from build123d import *

# Parameters (mm, degrees)
SKETCH1_W           = 4
SKETCH1_H           = 2
BOSS_EXTRUDE1_DEPTH = 3.5
WIRE_CANAL_DEPTH    = 1.5
SKETCH2_R           = 0.8
SCREW_HOLES_DEPTH   = 43.383720665
FILLET1_START       = 14.161255893
FILLET1_DEPTH       = 27.838744107
CUT_EXTRUDE1_START  = 3.5
SKETCH4_R           = 1.25
CUT_EXTRUDE1_DEPTH  = 3


with BuildPart() as part:
    # Sketch1 → Boss-Extrude1 (new body)
    with BuildSketch(Plane.XY):
        with BuildLine():
            Line((10.161255893, 0), (36.161255894, 0))
            ThreePointArc((36.161255894, 0), (37.476597455, 4.684658438), (41.038150268, 8))
            Line((41.038150268, 8), (14.161255893, 8))
            Line((14.161255893, 8), (10.161255893, 8))
            Line((10.161255893, 8), (10.161255893, 0))
        make_face()
        Polygon((36.161255894, -8), (36.161255894, 0), (10.161255893, 0), (10.161255893, -8), (14.161255893, -8), align=None)
        with Locations((12.161255893, 9)):
            Rectangle(SKETCH1_W, SKETCH1_H)
        with Locations((12.161255893, -9)):
            Rectangle(SKETCH1_W, SKETCH1_H)
    extrude(amount=BOSS_EXTRUDE1_DEPTH)

    # Sketch3 → Wire Canal (cut)
    with BuildSketch(Plane.XY):
        Polygon((10.161255893, 3), (10.161255893, 0), (10.161255893, -3), (38.287392351, -3), (38.287392351, 3), align=None)
    extrude(amount=WIRE_CANAL_DEPTH, mode=Mode.SUBTRACT)

    # Sketch2 → Screw Holes (cut, through all)
    with BuildSketch(Plane.XY):
        with Locations(Location((20.161255894, 0, 0), (0, 0, 180))):
            Circle(SKETCH2_R)
        with Locations((12.161255894, -6.25)):
            Circle(SKETCH2_R)
        with Locations((29.661255894, 6.25)):
            Circle(SKETCH2_R)
        with Locations((29.661255894, -6.25)):
            Circle(SKETCH2_R)
        with Locations((12.161255894, 6.25)):
            Circle(SKETCH2_R)
        with Locations(Location((28.161255894, 0, 0), (0, 0, 180))):
            Circle(SKETCH2_R)
    extrude(amount=SCREW_HOLES_DEPTH, mode=Mode.SUBTRACT)

    # Fillet1: read off the stored shape, not the designer's step
    # Fillet1 outline → Fillet1 (cut)
    with BuildSketch(Plane.YZ.offset(FILLET1_START)):
        with BuildLine():
            Line((-8, 3.5), (-8, 0.5))
            ThreePointArc((-8, 0.5), (-7.121320344, 2.621320344), (-5, 3.5))
            Line((-5, 3.5), (-8, 3.5))
        make_face()
        with BuildLine():
            Line((8, 3.5), (5, 3.5))
            ThreePointArc((5, 3.5), (7.121320344, 2.621320344), (8, 0.5))
            Line((8, 0.5), (8, 3.5))
        make_face()
    extrude(amount=FILLET1_DEPTH, mode=Mode.SUBTRACT)

    # Sketch4 → Cut-Extrude1 (cut)
    with BuildSketch(Plane.XY.offset(CUT_EXTRUDE1_START)):
        with Locations((29.661255894, -6.25)):
            Circle(SKETCH4_R)
    extrude(amount=-CUT_EXTRUDE1_DEPTH, mode=Mode.SUBTRACT)


solid = part.part
Source: CAD feature listing. Evaluate the final solid. Frame: model axes, mm. A direction names the side the tool comes from. Round coordinates to 2 decimals unless told otherwise and drop trailing zeros. Loops run counter-clockwise (first coordinate to the right, second up) from the corner with the lowest first, then second, coordinate; pieces in that order, holes last. Notation, with made-up numbers: M 4,-33 L 8,-33 A9 ccw 8,-19 Z; hole C 21.25,-11.5 d4. An arc over 180 degrees is marked long. Answer as CSV lines item,"result".
Q1. Contact query for flat-ended pins moving along their axis: pin 1 (1.8 mm diameter, centred on y = 7, z = 1.5, fed in from +X); pin 2 (1.4 mm diameter, centred on x = 29.66, y = 6.25, fed in from -Z); pin 3 (2 mm diameter, centred on x = 28.16, y = 0, fed in from -Z); pin 4 (1 mm diameter, centred on x = 32.5, z = 1.5, fed in from -Y). Output: stop coordinate, or through.
Verdict:
pin 1,"stops at x = 40.82"
pin 2,"passes through"
pin 3,"stops at z = 1.5"
pin 4,"stops at y = -7.96"
Q2. Cut plane A-A (x = 17). Return the cut outline in (y, z).
Verdict:
outline,"M -8,0 L -3,0 L -3,1.5 L 3,1.5 L 3,0 L 8,0 L 8,0.5 A3 ccw 5,3.5 L -5,3.5 A3 ccw -8,0.5 Z"
Q3. Cut plane D-D (y = -4.25). Return the cut outline in (x, z).
Verdict:
outline,"M 10.16,0 L 36.16,0 L 36.16,3.5 L 10.16,3.5 Z"
Q4. Cut plane B-B (y = 6.25). Return the cut outline in (x, z), plus the area to 3 significant figures.
Verdict:
outline,"M 10.16,0 L 11.36,0 L 11.36,3.5 L 10.16,3.5 Z; M 12.96,0 L 28.86,0 L 28.86,3.23 L 14.16,3.23 L 14.16,3.5 L 12.96,3.5 Z; M 30.46,0 L 38.69,0 L 38.69,3.23 L 30.46,3.23 Z"
area,"82.4 mm^2"
Q5. Reachability of faces 5 (the face through (36.161, -4, 2)), 6 (the face through (23, 0, 1.5)), 7 (the face through (11.57, 6.79, 1.73)) from +Z, -Z, +X, -X, +Y, -Y: full face, straight path, thin tool, end or side. Return the list, or none.
Verdict:
face 5,"+Z, -Z, +X, -Y"
face 6,"-Z, +X, -X"
face 7,"+Z, -Z"
Q6. Cut plane C-C (z = 2.85). Return the cut outline in (x, y), plus the area to 3 significant figures.
Verdict:
outline,"M 10.16,-10 L 14.16,-10 L 14.16,-6.86 L 28.57,-6.86 A1.25 cw long 30.75,-6.86 L 36.16,-6.86 L 36.16,0 A9 cw 39.34,6.86 L 30.17,6.86 A0.8 cw long 29.15,6.86 L 14.16,6.86 L 14.16,10 L 10.16,10 Z; hole C 12.16,-6.25 d1.6; hole C 12.16,6.25 d1.6; hole C 20.16,0 d1.6; hole C 28.16,0 d1.6"
area,"375 mm^2"
Q7. Line query: line 1 along X through (y, z) = (-6.25, 0.45); line 2 along X through (y, z) = (-6.25, 2.2); line 3 along Y through (x, z) = (13, 1). Output: solid intervals per line, ascending.
Verdict:
line 1,"x = 10.16 to 11.36, 12.96 to 28.86, 30.46 to 36.16"
line 2,"x = 10.16 to 11.36, 12.96 to 28.41, 30.91 to 36.16"
line 3,"y = -10 to -3, 3 to 10"
Q8. Pull-direction query (Y, two-part tool) for faces 1 (the face through (23, -3, 1)), 2 (the face through (14.161, -9, 2)), 3 (the face through (25.01, -7.14, 2.6)), 4 (the face through (29.5, -5.01, 1.69)); classes: +Y half, -Y half, draft (parallel to the pull), parting line (faces both ways), or undercut.
Verdict:
face 1,"undercut"
face 2,"draft"
face 3,"-Y half"
face 4,"undercut"
